For this review, take the finished solid that the model builds, in its own axes (mm). Face numbers are marked on the shaded views. A direction names the side the tool comes from. Round coordinates to 2 decimals unless told otherwise and drop trailing zeros. Write each loop counter-clockwise with the first axis right and the second up, starting at its lowest first coordinate (ties: lowest second). Pieces come first, ordered by that corner, then holes.
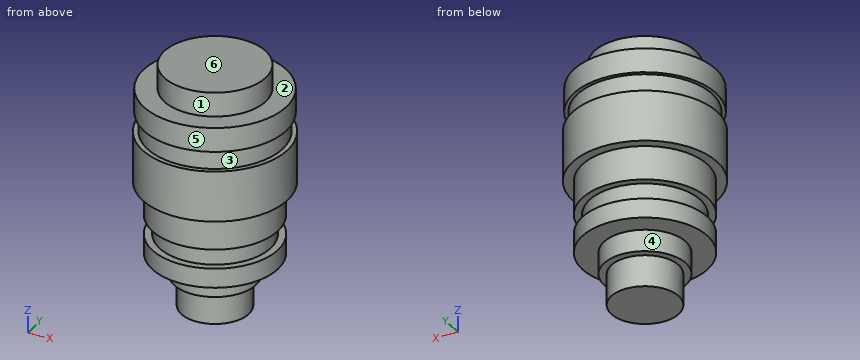
from build123d import *

# Parameters (mm, degrees)
SKETCH1_W   = 5
SKETCH1_H   = 10.5
SKETCH1_H_2 = 14.75
SKETCH1_W_2 = 4
SKETCH1_H_3 = 14
SKETCH1_H_4 = 11.5
SKETCH1_W_3 = 6.5
SKETCH1_H_5 = 7


with BuildPart() as part:
    # Sketch1 → Revolve1 (revolve)
    with BuildSketch(Plane(origin=(0, 0, 0), x_dir=(0, 0, -1), z_dir=(1, 0, 0)), mode=Mode.PRIVATE) as revolve1_sk:
        with Locations((-2.5, 5.25)):
            Rectangle(SKETCH1_W, SKETCH1_H)
        with Locations((2.5, 7.375)):
            Rectangle(SKETCH1_W, SKETCH1_H_2)
        with Locations((7, 7)):
            Rectangle(SKETCH1_W_2, SKETCH1_H_3)
        Polygon((9, 14), (9, 0), (19.5, 0), (19.5, 13), (19.5, 15), (9, 15), align=None)
        Polygon((19.5, 13), (19.5, 0), (26.5, 0), (26.5, 11.5), (26.5, 13), align=None)
        with Locations((28.5, 5.75)):
            Rectangle(SKETCH1_W_2, SKETCH1_H_4)
        Polygon((30.5, 11.5), (30.5, 0), (34.5, 0), (34.5, 8.5), (34.5, 13), (30.5, 13), align=None)
        Polygon((34.5, 8.5), (34.5, 0), (39, 0), (39, 7), (39, 8.5), align=None)
        with Locations((42.25, 3.5)):
            Rectangle(SKETCH1_W_3, SKETCH1_H_5)
    revolve(revolve1_sk.sketch.rotate(Axis((0, 0, -9), (0, 0, -1)), 90), axis=Axis((0, 0, -9), (0, 0, -1)))


solid = part.part
(1) For pin 1 Ø1 at (y, z) = (11.5, -26) entering from -X; pin 2 Ø10 at (y, z) = (-9, 0) entering from -X; pin 3 Ø12 at (y, z) = (-0.5, -30.5) entering from -X; pin 4 Ø13 at (x, y) = (-6, -4) entering from -Z, all flat-tipped, find the tip position at first contact; note any pin that passes through.
Geometry check:
pin 1: stops at x = -6.93
pin 2: stops at x = -14.2
pin 3: stops at x = -13
pin 4: stops at z = -45.5
(2) Mouldability with a two-part tool opening along Z and no side actions: class the marked faces 1, 2 and 3 as pulls with the +Z half, pulls with the -Z half, needs draft (parallel to the pull), parting line crosses it, or undercut.
Geometry check:
face 1: needs draft
face 2: pulls with the +Z half
face 3: undercut
(3) For line 1 along Z through (x, y) = (-12.5, -7); line 2 along Z through (x, y) = (2.5, 11); line 3 along Z through (x, y) = (6.25, 12), list the stretches that pass through material, from the lowest coordinate up.
Geometry check:
line 1: z = -19.5 to -9, -5 to 0
line 2: z = -34.5 to 0
line 3: z = -19.5 to 0
(4) We need section B-B, the plane z = -18.5. Give the boundary of the cut face in (x, y).
Geometry check:
outline: circle Ø30 at (0, 0)
(5) For the marked faces 4, 5 and 6, list the 3-axis set-ups (+Z, -Z, +X, -X, +Y, -Y) from which the entire face can be reached by the end or side of a thin tool; tool diameter is ignored.
Geometry check:
face 4: -Z
face 5: +Z
face 6: +Z, +X, -X, +Y, -Y
(6) We need section A-A, the plane z = -28.5. Give the boundary of the cut face in (x, y).
Geometry check:
outline: circle Ø23 at (0, 0)
